Autodesk Inventor part; units mm, degrees
ref_plane "Work Plane1" through (-17, 0, 0) normal (1, 0, 0) x (0, 0, -1)
ref_plane "Work Plane2" through (0, 80.8, 0) normal (0, 1, 0) x (1, 0, 0)
ref_plane "YZ Plane" through (0, 0, 0) normal (1, 0, 0) x (0, 1, 0)
sketch "Sketch1" plane through (0, 0, 0) normal (0, 1, 0) x (-1, 0, 0)
  line L0 (0, 0) -> (34, 0)
  line L1 (34, 0) -> (34, -80)
  line L2 (34, -80) -> (0, -80)
  line L3 (0, -80) -> (0, 0)
  dimension "d0" = 34
  dimension "d1" = 80
extrude "Extrusion1" add sketch "Sketch1" along normal blind 30
ref_plane "Work Plane1" through (-17, 0, 0) normal (1, 0, 0) x (0, 0, -1)
sketch "Sketch2" plane through (-17, 0, 0) normal (1, 0, 0) x (0, 0, -1)
  line L0 (80, 30) -> (0, 30)
  line L1 (40, 30) -> (27.3, 30)
  line L2 (40, 30) -> (52.7, 30)
  line L3 (52.7, 30) -> (55.7, 30)
  line L4 (80, 0) -> (80, 30)
  line L5 (80, 0) -> (79.25, 0)
  line L6 (80, 0) -> (0, 0)
  line L7 (79.25, 0) -> (55.7, 30)
  line L8 (27.3, 30) -> (24.3, 30)
  line L9 (0, 0) -> (0.75, 0)
  line L10 (0.75, 0) -> (24.3, 30)
  line L11 (0.75, 0) -> (79.25, 0)
  dimension "d4" = 12.7
  dimension "d5" = 12.7
  dimension "d6" = 3
  dimension "d7" = 0.75
  dimension "d8" = 3
  dimension "d9" = 0.75
extrude "Extrusion2" cut sketch "Sketch2" along normal mid plane 32.8 contours L7 L6 L10 L0
sketch "Sketch3" plane through (-34, 0, -80) normal (-1, 0, 0) x (0, 0, 1)
  line L0 (80, 30) -> (0, 30)
  line L1 (0, 0) -> (80, 0)
  line L2 (0, 30) -> (80, 30)
  line L3 (80, 30) -> (80, 0)
  line L4 (80, 0) -> (0, 0)
  line L5 (0, 0) -> (0, 30)
extrude "Extrusion3" add sketch "Sketch3" along normal blind 3
sketch "Sketch4" plane through (0, 0, 0) normal (1, 0, 0) x (0, 0, -1)
  line L0 (0, 0) -> (0, 30)
  line L1 (0, 0) -> (80, 0)
  line L2 (0, 30) -> (80, 30)
  line L3 (80, 30) -> (80, 0)
  line L4 (80, 0) -> (0, 0)
  line L5 (0, 0) -> (0, 30)
extrude "Extrusion4" add sketch "Sketch4" along normal blind 3
sketch "Sketch5" plane through (3, 0, 0) normal (1, 0, 0) x (0, 0, -1)
  line L0 (0, 30) -> (80, 30)
  line L1 (0, 30) -> (0, 20)
  line L2 (0, 0) -> (0, 30)
  line L3 (0, 30) -> (10, 30)
  line L4 (10, 30) -> (0, 20)
  line L5 (80, 30) -> (80, 0)
  line L6 (80, 30) -> (80, 20)
  line L7 (80, 30) -> (70, 30)
  line L8 (70, 30) -> (80, 20)
  dimension "d16" = 10
  dimension "d17" = 10
  dimension "d18" = 10
extrude "Extrusion5" cut sketch "Sketch5" against normal through all
sketch "Sketch6" plane through (0, 30, 0) normal (0, 1, 0) x (1, 0, 0)
  line L0 (-0.6, 24.3) -> (-33.4, 24.3)
  line L1 (-0.6, 55.7) -> (-0.6, 24.3)
  line L2 (-33.4, 24.3) -> (-0.6, 24.3)
  line L3 (-0.6, 24.3) -> (-0.6, 55.7)
  line L4 (-0.6, 55.7) -> (-33.4, 55.7)
  line L5 (-33.4, 55.7) -> (-33.4, 24.3)
  line L6 (-37, 20.7) -> (3, 20.7)
  line L7 (3, 20.7) -> (3, 59.3)
  line L8 (3, 59.3) -> (-37, 59.3)
  line L9 (-37, 59.3) -> (-37, 20.7)
  point P0 (0, 0)
  dimension "d21" = 3.6
extrude "Extrusion6" add sketch "Sketch6" along normal blind 76.2
sketch "Sketch7" plane through (3, 0, 0) normal (1, 0, 0) x (0, 0, -1)
  line L0 (20.7, 30) -> (10, 30)
  line L1 (10, 30) -> (20.7, 40.7)
  line L2 (20.7, 30) -> (20.7, 106.2)
  line L3 (10, 30) -> (25.1321, 30) construction
  line L4 (20.7, 40.7) -> (20.7, 30)
  line L5 (20.7, 30) -> (10, 30)
  line L6 (70, 30) -> (59.3, 30)
  line L7 (70, 30) -> (59.3, 40.7)
  line L8 (59.3, 30) -> (59.3, 106.2)
  line L9 (59.3, 40.7) -> (59.3, 30)
  line L10 (70, 30) -> (80, 20)
  line L11 (59.3, 30) -> (70, 30)
  point P0 (0, 0)
  dimension "d24" = 45
extrude "Extrusion7" add sketch "Sketch7" against normal up to surface (40 mm away)
ref_plane "Work Plane2" through (0, 80.8, 0) normal (0, 1, 0) x (1, 0, 0)
mirror "Mirror1" about plane through (0, 80.8, 0) normal (0, 1, 0)
properties part number "Bone_Cover"
Input: part model. Units: mm. Frame: model coordinates. A direction names the side the tool comes from. Round coordinates to 2 decimals unless told otherwise and drop trailing zeros. Loops run counter-clockwise (first coordinate to the right, second up) from the corner with the lowest first, then second, coordinate; pieces in that order, holes last. Notation, with made-up numbers: (86.5, 7) -> (145.5, 7) arc R16 ccw to (145.5, 31) -> close; hole circle Ø6 at (-21.5, 83). An arc over 180 degrees is marked (long way). Answer as a JSON object with one key per item and string values. Group by question number.
1) Pin query (flat end, axial travel): pin 1 (8 mm diameter, centred on x = -10, y = 136.5, fed in from -Z); pin 2 (1 mm diameter, centred on x = -6, y = 97, fed in from -Z); pin 3 (16.5 mm diameter, centred on x = -19, y = 71, fed in from +Z). Return the tip coordinate at first contact, or that it passes through.
2) Section query C-C on x = -17. Output: boundary loops of the cut face in (y, z).
3) Section query A-A on z = -51. Output: boundary loops of the cut face in (x, y).
4) Section query D-D on y = 57. Output: boundary loops of the cut face in (x, z), plus the area to 3 significant figures.
5) Draft query along Y for faces 4 (the flat face through (-33.4, 80, -41)), 5 (the flat face through (-16.7, 131.4, -10.2)), 6 (the flat face through (-17, 30, -10)), 7 (the flat face through (-17.23, 146.39, -12.69)). Return one class per face: +Y half, -Y half, draft (parallel to the pull), parting line (faces both ways), or undercut.
6) Reachability of faces 1 (the flat face through (-17, 80, -20.7)), 2 (the flat face through (-17, 80, -24.3)), 3 (the flat face through (-17, 30, -70)) from +Z, -Z, +X, -X, +Y, -Y: full face, straight path, thin tool, end or side. Return the list, or none.
7) Section query B-B on y = 129. Output: boundary loops of the cut face in (x, z), plus the area to 3 significant figures.
8) Ray query, L1, parallel to X at y = 44.5, z = -46.5; L2, parallel to Z at x = -16.5, y = 104; L3, parallel to Z at x = -15.5, y = 12.5. Return the intervals inside material, ascending.
Reply:
{
 "1": {"pin 1": "stops at z = -78.9", "pin 2": "stops at z = -59.3", "pin 3": "stops at z = -20.7"},
 "2": {"outline": "(0, -80) -> (20, -80) -> (40.7, -59.3) -> (120.9, -59.3) -> (141.6, -80) -> (161.6, -80) -> (161.6, -79.25) -> (131.6, -55.7) -> (30, -55.7) -> (0, -79.25) -> close; (0, -0.75) -> (30, -24.3) -> (131.6, -24.3) -> (161.6, -0.75) -> (161.6, 0) -> (141.6, 0) -> (120.9, -20.7) -> (40.7, -20.7) -> (20, 0) -> (0, 0) -> close"},
 "3": {"outline": "(-37, 0) -> (-33.4, 0) -> (-33.4, 161.6) -> (-37, 161.6) -> close; (-0.6, 0) -> (3, 0) -> (3, 161.6) -> (-0.6, 161.6) -> close"},
 "4": {"outline": "(-37, -59.3) -> (3, -59.3) -> (3, -20.7) -> (-37, -20.7) -> close; hole (-33.4, -55.7) -> (-0.6, -55.7) -> (-0.6, -24.3) -> (-33.4, -24.3) -> close", "area": "514 mm2"},
 "5": {"face 4": "draft", "face 5": "undercut", "face 6": "undercut", "face 7": "+Y half"},
 "6": {"face 1": "+Z, +X, -X", "face 2": "+Y, -Y", "face 3": "-Z, +X, -X"},
 "7": {"outline": "(-37, -67.4) -> (3, -67.4) -> (3, -12.6) -> (-37, -12.6) -> close; hole (-33.4, -55.7) -> (-0.6, -55.7) -> (-0.6, -24.3) -> (-33.4, -24.3) -> close", "area": "1,160 mm2"},
 "8": {"L1": "x = -37 to -33.4, -0.6 to 3", "L2": "z = -59.3 to -55.7, -24.3 to -20.7", "L3": "z = -80 to -69.44, -10.56 to 0"}
}
